Study the drawing (mm; zero at the part's minimum x, y, z) and answer. A direction names the side the tool comes from. Round coordinates to 2 decimals unless told otherwise and drop trailing zeros. Order: outer loops, then holes, each group sorted by start corner. A loop starts at its lowest first (then second) coordinate and runs counter-clockwise, first axis right, second up. Notation, with made-up numbers: (-16.5, 59) - (37.5, 59) arc R21 cw to (37.5, 82) - close; hole circle Ø4 at (48.25, 15.25). An arc over 180 degrees is marked (long way). Put each result on its own line as item: value.
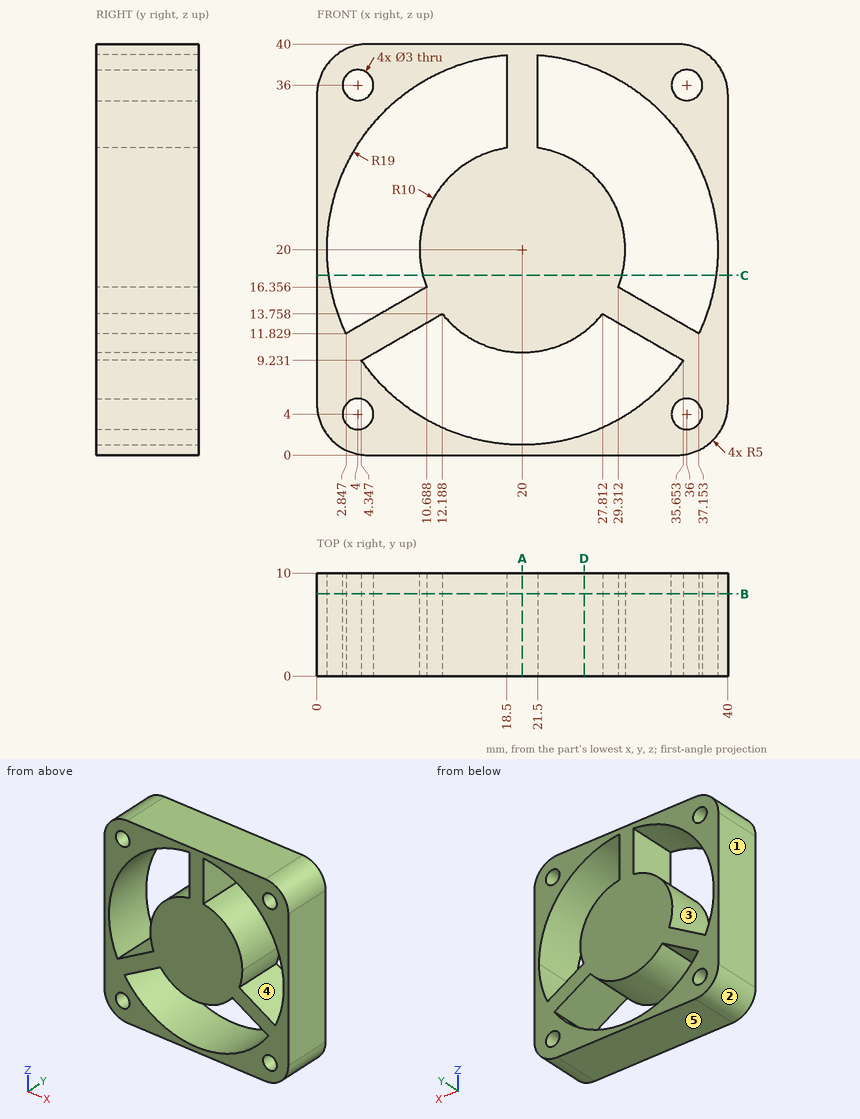
1) For a pull along Z with two mould halves and no side action, classify the marked faces 1, 2 and 3 as pulls with the +Z half, pulls with the -Z half, needs draft (parallel to the pull), parting line crosses it, or undercut.
Findings below:
face 1: needs draft
face 2: pulls with the -Z half
face 3: undercut
2) A cutting plane is placed at D-D on x = 26. Write down the section's boundary in (y, z).
Findings below:
outline: (0, 0) - (10, 0) - (10, 1.97) - (0, 1.97) - close; (0, 12) - (10, 12) - (10, 28) - (0, 28) - close; (0, 38.03) - (10, 38.03) - (10, 40) - (0, 40) - close
3) A cutting plane is placed at A-A on x = 20. Write down the section's boundary in (y, z).
Findings below:
outline: (0, 0) - (10, 0) - (10, 1) - (0, 1) - close; (0, 10) - (10, 10) - (10, 40) - (0, 40) - close
4) Straight lines are drawn through the part: L1, parallel to Z at x = 31, y = 0.5 (1 decimal); L2, parallel to X at y = 4.5, z = 15.5 (1 decimal); L3, parallel to Z at x = 14, y = 9.25. For each, find the intervals that lie inside material, in ascending order. Write a range as from..to.
Findings below:
L1: z = 0..4.5, 11.9..15.4, 35.5..40
L2: x = 0..1.5, 9.2..30.8, 38.5..40
L3: z = 0..1.97, 12..28, 38.03..40
5) Given pin 1 Ø2.5 at (y, z) = (6, 36.5) entering from -X; pin 2 Ø5 at (x, z) = (28, 31) entering from +Y, each flat-ended and moving along its own axis, determine where each tip first touches the part or whether it passes through.
Findings below:
pin 1: stops at x = 0.01
pin 2: passes through
6) A cutting plane is placed at C-C on z = 17.5. Write down the section's boundary in (x, y) (1 decimal), then the cut area to 3 significant figures.
Findings below:
outline: (0, 0) - (1.2, 0) - (1.2, 10) - (0, 10) - close; (10.3, 0) - (29.7, 0) - (29.7, 10) - (10.3, 10) - close; (38.8, 0) - (40, 0) - (40, 10) - (38.8, 10) - close
area: 217 mm2
7) A cutting plane is placed at B-B on y = 8. Write down the section's boundary in (x, z) (1 decimal).
Findings below:
outline: (0, 5) arc R5 ccw to (5, 0) - (35, 0) arc R5 ccw to (40, 5) - (40, 35) arc R5 ccw to (35, 40) - (5, 40) arc R5 ccw to (0, 35) - close; hole circle Ø3 at (4, 4); hole circle Ø3 at (4, 36); hole (2.8, 11.8) - (10.7, 16.4) arc R10 cw to (18.5, 29.9) - (18.5, 38.9) arc R19 ccw to start; hole (4.3, 9.2) arc R19 ccw to (35.7, 9.2) - (27.8, 13.8) arc R10 cw to (12.2, 13.8) - close; hole (21.5, 29.9) arc R10 cw to (30, 20) arc R10 cw to (29.3, 16.4) - (37.2, 11.8) arc R19 ccw to (39, 20) arc R19 ccw to (21.5, 38.9) - close; hole circle Ø3 at (36, 4); hole circle Ø3 at (36, 36)
8) For the marked faces 4 and 5, determine the directions among +Z, -Z, +X, -X, +Y, -Y from which every point of the face is accessible in a straight line to the end or side of a thin tool.
Findings below:
face 4: +Y, -Y
face 5: -Z, +X, -X, +Y, -Y
